Here's the drawing with two shaded views (mm, measured from the low corner). I have some questions. Round coordinates to 2 decimals unless told otherwise and drop trailing zeros. Write each loop counter-clockwise with the first axis right and the second up, starting at its lowest first coordinate (ties: lowest second). Pieces come first, ordered by that corner, then holes. Notation, with made-up numbers: M 58,-24 L 115,-24 A30 cw 115,13 Z; hole C 38.25,63 d1. An arc over 180 degrees is marked long. Answer as a JSON object with one key per item and string values. Group by question number.
1) Please list where these lines run through material, in increasing order: L1, parallel to X at y = 44, z = 0.2; L2, parallel to Y at x = 157, z = 1.8; L3, parallel to X at y = 8, z = 0.75. Write a range as [from, to].
2) Suppose I cut it at C-C, the plane x = 101. Write out the boundary of the cut face in (y, z).
3) Suppose I cut it at A-A, the plane z = 2.65. Write out the boundary of the cut face in (x, y).
4) Suppose I cut it at B-B, the plane y = 19. Write out the boundary of the cut face in (x, z), and give its area (3 significant figures).
5) I'm going to push a flat-ended pin straight in: pin 1 Ø12 at (x, y) = (114.5, 58.5) entering from -Z. Where does the tip first touch, or does it pass through?
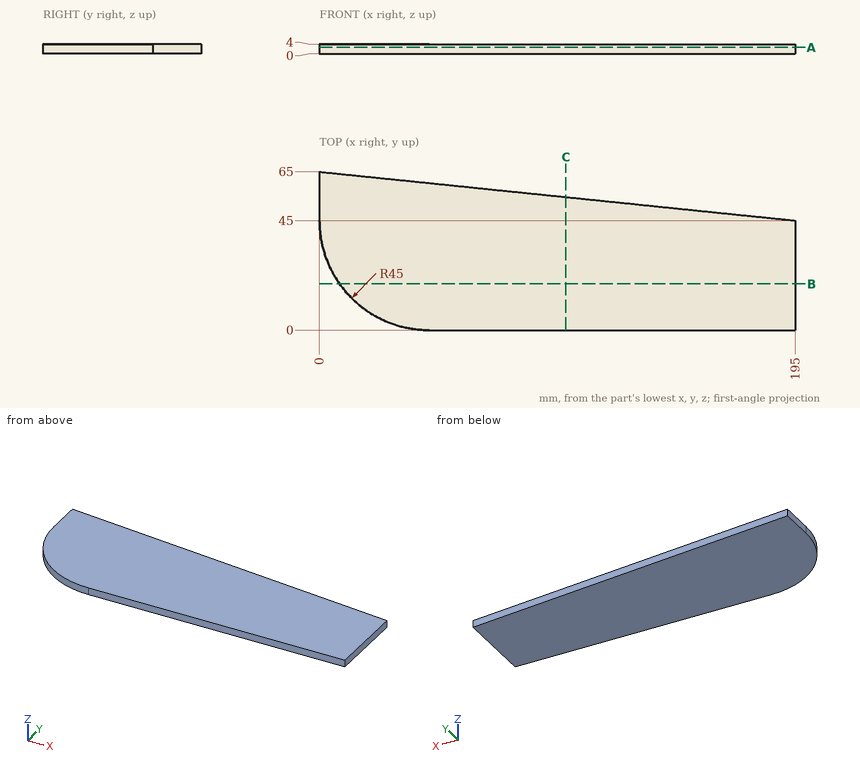
Results:
{
 "1": {"L1": "[0.01, 195]", "L2": "[0, 48.9]", "L3": "[19.39, 195]"},
 "2": {"outline": "M 0,0 L 54.64,0 L 54.64,4 L 0,4 Z"},
 "3": {"outline": "M 0,45 A45 ccw 45,0 L 195,0 L 195,45 L 0,65 Z"},
 "4": {"outline": "M 8.27,0 L 195,0 L 195,4 L 8.27,4 Z", "area": "747 mm^2"},
 "5": {"pin 1": "z = 0"}
}
